For this review, take the finished solid that the model builds, in its own axes (mm). Round coordinates to 2 decimals unless told otherwise and drop trailing zeros. Loops run counter-clockwise (first coordinate to the right, second up) from the corner with the lowest first, then second, coordinate; pieces in that order, holes last.
1. Consider section D-D on z = 40. State the section outline as (x, y) points, then the cut area to 3 significant figures.
2. Clearance check with flat-ended pins moving along their axes: pin 1 Ø3 at (x, z) = (-19, 37) entering from -Y; pin 2 Ø1 at (y, z) = (0.5, 11) entering from -X; pin 3 Ø2 at (y, z) = (0.5, -24.5) entering from +X; pin 4 Ø1.6 at (x, y) = (3.5, 1) entering from -Z. State where each tip first meets the part, or that it passes through.
3. To check wall thickness, follow line 1 along X through (y, z) = (2.4, -53.5); line 2 along X through (y, z) = (1.15, 53.5); line 3 along Z through (x, y) = (15, 1.95). State the ranges of each line that lie inside material, in increasing order.
4. Consider section C-C on x = -28.5. State the section outline as (y, z) points.
5. Consider section B-B on y = 0.65. State the section outline as (x, z) points, then the cut area to 3 significant figures.
6. Consider section A-A on z = -53.5. State the section outline as (x, y) points, then the cut area to 3 significant figures.
from build123d import *

# Parameters (mm, degrees)
SKETCH_1_W          = 64
SKETCH_1_H          = 114
EXTRUDE_1_DEPTH     = 2
SKETCH_2_W          = 70
SKETCH_2_H          = 120
EXTRUDE_4_DEPTH     = 2
SKETCH_4_R          = 1.4
CUT_EXTRUDE_1_DEPTH = 70.577295147


with BuildPart() as part:
    # Эскиз1 → Бобышка-Вытянуть1 (new body)
    with BuildSketch(Plane(origin=(0, 0, 0), x_dir=(1, 0, 0), z_dir=(0, 1, 0))):
        Rectangle(SKETCH_1_W, SKETCH_1_H)
    extrude(amount=EXTRUDE_1_DEPTH)

    # Эскиз2 → Бобышка-Вытянуть4 (add)
    with BuildSketch(Plane(origin=(0, 2, 0), x_dir=(1, 0, 0), z_dir=(0, 1, 0))):
        Rectangle(SKETCH_2_W, SKETCH_2_H)
    extrude(amount=EXTRUDE_4_DEPTH)

    # Эскиз4 → Вырез-Вытянуть1 (cut, through all)
    with BuildSketch(Plane(origin=(0, 4, 0), x_dir=(1, 0, 0), z_dir=(0, 1, 0))):
        with Locations(Location((-28.5, 53.5, 0), (0, 0, 270))):
            Circle(SKETCH_4_R)
        with Locations(Location((28.5, 53.5, 0), (0, 0, 270))):
            Circle(SKETCH_4_R)
        with Locations(Location((-28.5, -53.5, 0), (0, 0, 270))):
            Circle(SKETCH_4_R)
        with Locations(Location((28.5, -53.5, 0), (0, 0, 270))):
            Circle(SKETCH_4_R)
    extrude(amount=-CUT_EXTRUDE_1_DEPTH, mode=Mode.SUBTRACT)


solid = part.part
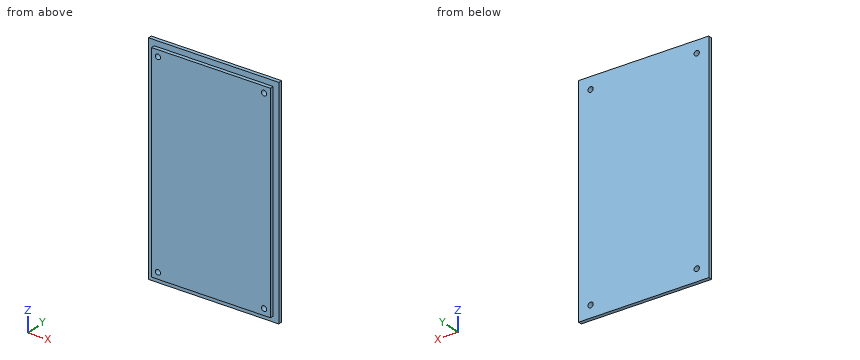
Resolved:
1. outline: (-35, 2) - (-32, 2) - (-32, 0) - (32, 0) - (32, 2) - (35, 2) - (35, 4) - (-35, 4) - close
1. area: 268 mm2
2. pin 1: stops at y = 0
2. pin 2: stops at x = -32
2. pin 3: stops at x = 32
2. pin 4: stops at z = -57
3. line 1: x = -35 to -29.9, -27.1 to 27.1, 29.9 to 35
3. line 2: x = -32 to -29.9, -27.1 to 27.1, 29.9 to 32
3. line 3: z = -57 to 57
4. outline: (0, -57) - (2, -57) - (2, -60) - (4, -60) - (4, -54.9) - (0, -54.9) - close; (0, -52.1) - (4, -52.1) - (4, 52.1) - (0, 52.1) - close; (0, 54.9) - (4, 54.9) - (4, 60) - (2, 60) - (2, 57) - (0, 57) - close
5. outline: (-32, -57) - (32, -57) - (32, 57) - (-32, 57) - close; hole circle Ø2.8 at (-28.5, -53.5); hole circle Ø2.8 at (-28.5, 53.5); hole circle Ø2.8 at (28.5, -53.5); hole circle Ø2.8 at (28.5, 53.5)
5. area: 7,270 mm2
6. outline: (-35, 2) - (-32, 2) - (-32, 0) - (-29.9, 0) - (-29.9, 4) - (-35, 4) - close; (-27.1, 0) - (27.1, 0) - (27.1, 4) - (-27.1, 4) - close; (29.9, 0) - (32, 0) - (32, 2) - (35, 2) - (35, 4) - (29.9, 4) - close
6. area: 246 mm2
